Autodesk Inventor part; units mm, degrees
ref_plane "YZ Plane" through (0, 0, 0) normal (1, 0, 0) x (0, 1, 0)
ref_plane "XZ Plane" through (0, 0, 0) normal (0, 1, 0) x (-1, 0, 0)
ref_plane "XY Plane" through (0, 0, 0) normal (0, 0, 1) x (1, 0, 0)
sketch "Face" plane through (0, 0, 0) normal (0, 0, 1) x (1, 0, 0)
  circle A0 centre (165.25, 188.4851) radius 2.6
  line L0 (158.2922, 98.7156) -> (160.7871, 98.7156)
  line L1 (160.7871, 92.4666) -> (158.965, 92.4666)
  arc A1 (158.965, 92.4666) -> (155.1773, 89.7524) centre (158.965, 88.4666) ccw
  circle A2 centre (114.75, 121.9851) radius 1.4
  arc A3 (154.6425, 101.0786) -> (155.1773, 89.7524) centre (140.5, 94.7351) ccw
  circle A4 centre (166.25, 70.4851) radius 1.4
  circle A5 centre (66.134, 121.9851) radius 1.4
  circle A6 centre (49.495, 121.2351) radius 2
  line L2 (180, 0) -> (180, 240.4851)
  line L3 (0, 0) -> (0, 240.4851)
  circle A7 centre (49.495, 96.2351) radius 16
  circle A8 centre (66.134, 70.4851) radius 1.4
  circle A9 centre (47.0211, 71.2351) radius 2
  line L4 (0, 0) -> (180, 0)
  circle A10 centre (90, 10) radius 2.6
  circle A11 centre (14.634, 121.9851) radius 1.4
  arc A12 (154.6425, 101.0786) -> (158.2922, 98.7156) centre (158.2922, 102.7156) ccw
  circle A13 centre (14.75, 52) radius 2.6
  circle A14 centre (90, 230.4851) radius 2.6
  circle A15 centre (14.75, 188.4851) radius 2.6
  circle A16 centre (165.25, 52) radius 2.6
  line L5 (180, 240.4851) -> (0, 240.4851)
  circle A17 centre (166.25, 121.9851) radius 1.4
  circle A18 centre (14.634, 70.4851) radius 1.4
  arc A19 (160.7871, 92.4666) -> (160.7871, 98.7156) centre (160.7871, 95.5911) ccw
  circle A20 centre (114.75, 70.4851) radius 1.4
  point P0 (106.7876, 102.9578)
sketch "PEEP Cutout" plane through (0, 0, 0) normal (0, 0, 1) x (1, 0, 0)
  circle A0 centre (66.134, -170) radius 1.4
  circle A1 centre (66.134, -118.5) radius 1.4
  arc A2 (52.8678, -166.7992) -> (55.0778, -122.1441) centre (49.495, -144.25) ccw
  arc A3 (52.8678, -166.7992) -> (50.5689, -169.3746) centre (53.2672, -169.4694) ccw
  arc A4 (43.5176, -168.6769) -> (50.5689, -169.3746) centre (47.0211, -169.25) ccw
  arc A5 (43.5176, -168.6769) -> (41.7681, -165.7008) centre (40.8531, -168.241) ccw
  arc A6 (43.9122, -122.1441) -> (41.7681, -165.7008) centre (49.495, -144.25) ccw
  arc A7 (43.9122, -122.1441) -> (45.9485, -119.4069) centre (43.2511, -119.5262) ccw
  arc A8 (53.0415, -119.4069) -> (45.9485, -119.4069) centre (49.495, -119.25) ccw
  arc A9 (53.0415, -119.4069) -> (55.0778, -122.1441) centre (55.7389, -119.5262) ccw
  circle A10 centre (14.634, -170) radius 1.4
  circle A11 centre (14.634, -118.5) radius 1.4
  point P0 (46.7949, -144.2181)
sketch "Sketch1" plane through (0, 0, 0) normal (0, 0, 1) x (1, 0, 0)
  circle A0 centre (75.25, 68.2425) radius 2.6
  line L0 (68.2922, -21.527) -> (70.7871, -21.527)
  line L1 (70.7871, -27.776) -> (68.965, -27.776)
  arc A1 (68.965, -27.776) -> (65.1773, -30.4901) centre (68.965, -31.776) ccw
  circle A2 centre (24.75, 1.7425) radius 1.4
  arc A3 (64.6425, -19.164) -> (65.1773, -30.4901) centre (50.5, -25.5075) ccw
  circle A4 centre (76.25, -49.7575) radius 1.4
  circle A5 centre (-23.866, 1.7425) radius 1.4
  circle A6 centre (-40.505, 0.9925) radius 2
  line L2 (90, -120.2425) -> (90, 120.2425)
  line L3 (-90, -120.2425) -> (-90, 120.2425)
  circle A7 centre (-40.505, -24.0075) radius 16
  circle A8 centre (-23.866, -49.7575) radius 1.4
  circle A9 centre (-42.9789, -49.0075) radius 2
  line L4 (-90, -120.2425) -> (90, -120.2425)
  circle A10 centre (0, -110.2425) radius 2.6
  circle A11 centre (-75.366, 1.7425) radius 1.4
  arc A12 (64.6425, -19.164) -> (68.2922, -21.527) centre (68.2922, -17.527) ccw
  circle A13 centre (-75.25, -68.2425) radius 2.6
  circle A14 centre (0, 110.2425) radius 2.6
  circle A15 centre (-75.25, 68.2425) radius 2.6
  circle A16 centre (75.25, -68.2425) radius 2.6
  line L5 (90, 120.2425) -> (-90, 120.2425)
  circle A17 centre (76.25, 1.7425) radius 1.4
  circle A18 centre (-75.366, -49.7575) radius 1.4
  arc A19 (70.7871, -27.776) -> (70.7871, -21.527) centre (70.7871, -24.6515) ccw
  circle A20 centre (24.75, -49.7575) radius 1.4
  point P0 (0, 0)
  point P1 (90, 0)
  point P2 (0, -120.2425)
extrude "Extrusion1" add sketch "Sketch1" along normal mid plane 4.75
sketch "Sketch2" plane through (0, 0, 2.375) normal (0, 0, 1) x (1, 0, 0)
  circle A0 centre (0, 110.2425) radius 2.6
  circle A1 centre (0, -110.2425) radius 2.6
  point P0 (0, 0)
  point P1 (46.8313, 110.2425)
  point P2 (-46.8312, 110.2425)
  point P3 (-46.8312, -110.2425)
  point P4 (46.8313, 110.2425)
  point P5 (46.8313, -110.2425)
  dimension "d2" = 93.6625
  dimension "d3" = 46.8312
hole "Hole1" at (46.8313, 110.2425, 2.375) at (-46.8312, 110.2425, 2.375) at (-46.8312, -110.2425, 2.375) at (46.8313, -110.2425, 2.375) direction (0, 0, -1) diameter 5.5 end through all
sketch "Sketch3" plane through (0, 0, 2.375) normal (0, 0, 1) x (1, 0, 0)
  circle A0 centre (-40.505, -24.0075) radius 16
  circle A1 centre (-23.866, -49.7575) radius 1.4
  circle A2 centre (-23.866, -49.7575) radius 1.4
  circle A3 centre (-23.866, 1.7425) radius 1.4
  arc A4 (-37.1322, -46.5566) -> (-34.9222, -1.9015) centre (-40.505, -24.0075) ccw
  arc A5 (-37.1322, -46.5566) -> (-39.4311, -49.1321) centre (-36.7328, -49.2269) ccw
  arc A6 (-46.4824, -48.4343) -> (-39.4311, -49.1321) centre (-42.9789, -49.0075) ccw
  arc A7 (-46.4824, -48.4343) -> (-48.2319, -45.4582) centre (-49.1469, -47.9984) ccw
  arc A8 (-46.0878, -1.9015) -> (-48.2319, -45.4582) centre (-40.505, -24.0075) ccw
  arc A9 (-46.0878, -1.9015) -> (-44.0515, 0.8356) centre (-46.7489, 0.7163) ccw
  arc A10 (-36.9585, 0.8356) -> (-44.0515, 0.8356) centre (-40.505, 0.9925) ccw
  arc A11 (-36.9585, 0.8356) -> (-34.9222, -1.9015) centre (-34.2611, 0.7163) ccw
  circle A12 centre (-75.366, -49.7575) radius 1.4
  circle A13 centre (-75.366, 1.7425) radius 1.4
  point P0 (0, 0)
extrude "Extrusion2" cut sketch "Sketch3" against normal through all contours A5 A6 A7 A8 A9 A10 A11 A4
properties part number "BREEZE-M10"
CAD build for the part. Positions are in the model's coordinates, mm. A direction names the side the tool comes from. Coordinates: 2 decimals unless noted, no trailing zeros. Write each loop counter-clockwise with the first axis right and the second up, starting at its lowest first coordinate (ties: lowest second). Pieces come first, ordered by that corner, then holes.
(1) 3-axis set-ups, long thin cutter, end or side, ignore diameter. For faces 1 (the face through (-17.76, -25.57, 0.03)), 2 (the face through (1, 120.242, 0)): which of +Z, -Z, +X, -X, +Y, -Y reach the whole face in a straight line?
(2) Cut at A-A, the plane x = 0. List the corners of the cut face in (y, z) (1 decimal), and give its area (3 significant figures).
(3) Drill centre lines: probe 1 along Y at (x, z) = (24.75, -1.25); probe 2 along Y at (x, z) = (24.5, 1.5) (1 decimal); probe 3 along X at (y, z) = (-68.5, -1). Where is each one in solid material? Low to high.
(4) Two-plate mould, pull along Y, no slides. Class faces 3 (the face through (-1, 2, 2.375)), 4 (the face through (46.005, -112.866, -0.033)), 5 (the face through (-1, -120.242, 0)): +Y half, -Y half, draft (parallel to the pull), parting line (faces both ways), or undercut.
(5) Cut at B-B, the plane z = -0.15. Count the separate pieces of the cut face and the enclosed holes in it, and give its area (3 significant figures).
(6) Flat gauge pin, fed straight in: pin 1 (3 mm diameter, centred on x = 76.25, y = -49.76, fed in from +Z) (3 decimals). Where does the tip first touch, or does it go through?
Geometry says:
1. face 1: +Z, -Z
1. face 2: +Z, -Z, +X, -X, +Y
2. outline: (-120.2, -2.4) - (-112.8, -2.4) - (-112.8, 2.4) - (-120.2, 2.4) - close; (-107.6, -2.4) - (107.6, -2.4) - (107.6, 2.4) - (-107.6, 2.4) - close; (112.8, -2.4) - (120.2, -2.4) - (120.2, 2.4) - (112.8, 2.4) - close
2. area: 1,090 mm2
3. probe 1: y = -120.24 to -51.16, -48.36 to 0.34, 3.14 to 120.24
3. probe 2: y = -120.2 to -51.1, -48.4 to 0.4, 3.1 to 120.2
3. probe 3: x = -90 to -77.84, -72.66 to 72.66, 77.84 to 90
4. face 3: draft
4. face 4: undercut
4. face 5: -Y half
5. separate pieces: 1
5. enclosed holes: 20
5. area: 40,500 mm2
6. pin 1: stops at z = 2.375
